```python
from build123d import *

# Parameters (mm, degrees)
SKETCH1_R                = 2.5
BOSS_EXTRUDE1_DEPTH      = 4
SKETCH1_3_R              = 5
BOSS_EXTRUDE2_DEPTH      = 1
BOSS_EXTRUDE3_DEPTH      = 6
BOSS_EXTRUDE3_DEPTH_BACK = 28
BOSS_EXTRUDE3_START      = -1
SKETCH1_4_R              = 5
SKETCH1_4_R_2            = 3
SKETCH2_R                = 5
BOSS_EXTRUDE6_DEPTH      = 2
BOSS_EXTRUDE7_DEPTH      = 5
BOSS_EXTRUDE7_DEPTH_BACK = 3
SKETCH2_5_R              = 2.5
CHAMFER1_SIZE            = 1


with BuildPart() as part:
    # Sketch1 → Boss-Extrude1 (new, symmetric)
    with BuildSketch(Plane.YZ):
        with Locations(Location((13.5, -14.43, 0), (0, 0, 270))):
            Circle(SKETCH1_R)
    extrude(amount=BOSS_EXTRUDE1_DEPTH, both=True)

    # Sketch1<3> → Boss-Extrude2 (add, symmetric)
    with BuildSketch(Plane.YZ):
        with BuildLine():
            Line((15.666598525, -13.182662503), (6.06647587, 3.492544992))
            ThreePointArc((6.06647587, 3.492544992), (-6.939551113, 0.917948988), (4.949747468, -4.949747468))
            ThreePointArc((4.949747468, -4.949747468), (8.491768153, -9.35999415), (11, -14.43))
            ThreePointArc((11, -14.43), (12.854436801, -12.014788176), (15.666598525, -13.182662503))
        make_face()
        with Locations(Location((0, 0, 0), (0, 0, 270))):
            Circle(SKETCH1_3_R, mode=Mode.SUBTRACT)
    extrude(amount=BOSS_EXTRUDE2_DEPTH, both=True)

    # Sketch1<4> → Boss-Extrude3 (add, two sides: drawn at the far end of the back side and taken through both)
    with BuildSketch(Plane.YZ.offset(BOSS_EXTRUDE3_START - BOSS_EXTRUDE3_DEPTH_BACK)):
        with Locations(Location((0, 0, 0), (0, 0, 270))):
            Circle(SKETCH1_4_R)
        with Locations(Location((0, 0, 0), (0, 0, 270))):
            Circle(SKETCH1_4_R_2, mode=Mode.SUBTRACT)
    extrude(amount=BOSS_EXTRUDE3_DEPTH + BOSS_EXTRUDE3_DEPTH_BACK)

    # Sketch2 → Boss-Extrude6 (add)
    # profile 1 of 2: a face of its own
    with BuildSketch(Plane(origin=(-23, 0, 0), x_dir=(0, -1, 0), z_dir=(-1, 0, 0))):
        with BuildLine():
            ThreePointArc((-9.4233e-05, 6.999999999), (-3.50376631, 6.060001786), (-6.06647587, 3.492544992))
            Line((-6.06647587, 3.492544992), (-15.666598525, -13.182662503))
            ThreePointArc((-15.666598525, -13.182662503), (-12.854436801, -12.014788176), (-11, -14.43))
            ThreePointArc((-11, -14.43), (-8.491768153, -9.35999415), (-4.949747468, -4.949747468))
            ThreePointArc((-4.949747468, -4.949747468), (2.678784027, -6.467156728), (7, 0))
            ThreePointArc((7, 0), (4.949714152, 4.949780784), (-9.4233e-05, 6.999999999))
        make_face()
        with Locations(Location((0, 0, 0), (0, 0, 270))):
            Circle(SKETCH2_R, mode=Mode.SUBTRACT)
    # profile 2 of 2: a face of its own
    with BuildSketch(Plane(origin=(-23, 0, 0), x_dir=(0, -1, 0), z_dir=(-1, 0, 0))):
        with BuildLine():
            ThreePointArc((22.5, -0.03), (11.786311318, 5.201659363), (-9.4233e-05, 6.999999999))
            ThreePointArc((-9.4233e-05, 6.999999999), (4.949714152, 4.949780784), (7, 0))
            ThreePointArc((7, 0), (13.62196533, -0.638300674), (20, -2.53))
            ThreePointArc((20, -2.53), (20.732233047, -0.762233047), (22.5, -0.03))
        make_face()
    extrude(amount=BOSS_EXTRUDE6_DEPTH)

    # Sketch2<5> → Boss-Extrude7 (add, two sides: drawn at the far end of the back side and taken through both)
    with BuildSketch(Plane(origin=(-23, 0, 0), x_dir=(0, -1, 0), z_dir=(-1, 0, 0)).offset(-BOSS_EXTRUDE7_DEPTH_BACK)):
        with Locations(Location((22.5, -2.53, 0), (0, 0, 90))):
            Circle(SKETCH2_5_R)
        with Locations(Location((-13.5, -14.43, 0), (0, 0, 270))):
            Circle(SKETCH2_5_R)
    extrude(amount=BOSS_EXTRUDE7_DEPTH + BOSS_EXTRUDE7_DEPTH_BACK)

    # Chamfer1
    chamfer1_edges = [part.edges().sort_by_distance(p)[0] for p in [
        (-29, 0, 5),
        (5, 0, 5),
    ]]
    chamfer(chamfer1_edges, length=CHAMFER1_SIZE)


solid = part.part
```
Build history of the part. All positions in model axes, mm. A direction names the side the tool comes from. Coordinates: 2 decimals unless noted, no trailing zeros. Order: outer loops, then holes, each group sorted by start corner. A loop starts at its lowest first (then second) coordinate and runs counter-clockwise, first axis right, second up. Notation, with made-up numbers: (11, -18.75) -> (29, -18.75) arc R14 cw to (29, -0.75) -> close; hole circle Ø2 at (-8.5, 83). An arc over 180 degrees is marked (long way). Answer in a Markdown table with one row per item. Add a question column.
Q1. Mould opens along Y. For faces 4 (the face through (-23.986, 3.459, 6.086)), 5 (the face through (-23.944, -24.021, -4.514)), 6 (the face through (5, 3, -1)) say: +Y half, -Y half, draft (parallel to the pull), parting line (faces both ways), or undercut.
Q2. Band-saw the part on A-A, the plane x = -24.5. List the corners of the cut face in (y, z).
Q3. Band-saw the part on C-C, the plane x = -11. List the corners of the cut face in (y, z), then the cut area to 3 significant figures.
Q4. Band-saw the part on B-B, the plane z = -8. List the corners of the cut face in (x, y), then the cut area to 3 significant figures.
Q5. Drop flat-ended pins along their axis: pin 1 (12 mm diameter, centred on y = -4.5, z = -14, fed in from -X); pin 2 (5 mm diameter, centred on x = 0, y = 4, fed in from +Z); pin 3 (5.5 mm diameter, centred on y = 13, z = -14.5, fed in from +X); pin 4 (12 mm diameter, centred on x = -5, y = -3, fed in from -Z). Give the stop position or say it passes through.
Q6. Wall check: line 1 along Y through (x, z) = (-20.5, 0); line 2 along X through (y, z) = (2.5, -4.75); line 3 along X through (y, z) = (-14, 2). Give the ranges that are in metal, low to high. Write a range as [from, to].
Q7. Which spindle directions (+Z, -Z, +X, -X, +Y, -Y) get a long thin tool onto all of the face, cutting with end or side? Do faces 1 (the face through (-20, -22, -3)), 2 (the face through (-23.99, -13.53, -0.62)), 3 (the face through (2.48, -4.88, 1.08)). Say none if no direction does.
Answers follow:
| question | item | result |
|---|---|---|
| 1 | face 4 | +Y half |
| 1 | face 5 | undercut |
| 1 | face 6 | draft |
| 2 | outline | (-22.5, -0.03) arc R2.5 ccw (long way) to (-20, -2.53) arc R34.66 cw to (-7, 0) arc R7 ccw to (4.95, -4.95) arc R26.09 cw to (11, -14.43) arc R2.5 ccw (long way) to (15.67, -13.18) -> (6.07, 3.49) arc R7 ccw to (0, 7) arc R39.52 ccw to start; hole circle Ø6 at (0, 0) |
| 3 | outline | circle Ø10 at (0, 0); hole circle Ø6 at (0, 0) |
| 3 | area | 50.3 mm^2 |
| 4 | outline | (-25, 7.56) -> (-23, 7.56) -> (-23, 12.68) -> (-25, 12.68) -> close; (-1, 7.56) -> (1, 7.56) -> (1, 12.68) -> (-1, 12.68) -> close |
| 4 | area | 20.5 mm^2 |
| 5 | pin 1 | through |
| 5 | pin 2 | z = 6.84 |
| 5 | pin 3 | x = 4 |
| 5 | pin 4 | z = -7 |
| 6 | line 1 | [-5, -3], [3, 5] |
| 6 | line 2 | [-25, -23], [-1, 1] |
| 6 | line 3 | [-25, -23] |
| 7 | face 1 | +Z, -Z, +X, -Y |
| 7 | face 2 | -Z, +X, -X |
| 7 | face 3 | +X |
